Geometry check sheet. Reference: the model listing, model coordinates, mm. Face numbers are marked on the shaded views. A direction names the side the tool comes from. Round coordinates to 2 decimals unless told otherwise and drop trailing zeros. Order: outer loops, then holes, each group sorted by start corner. A loop starts at its lowest first (then second) coordinate and runs counter-clockwise, first axis right, second up.
(1) Cross-section at A-A on y = 20. Enter the section's corners in (x, z).
(2) Cross-section at B-B on x = 0. Enter the section's corners in (y, z).
(3) Set-up check for the marked faces 4, 5 and 6: record each of +Z, -Z, +X, -X, +Y, -Y from which the full face is reachable in a straight line by a thin tool's end or side.
(4) Thickness scan on L1, parallel to Y at x = -17, z = 0; L2, parallel to X at y = 50, z = 0; L3, parallel to Z at x = -17.5, y = 20. Record the ranges inside material, lowest first.
(5) Cross-section at D-D on z = 17. Enter the section's corners in (x, y).
(6) Draft check along Z on the marked faces 1, 2 and 3. Enter one of: pulls with the +Z half, pulls with the -Z half, needs draft (parallel to the pull), parting line crosses it, or undercut.
(7) Gauge pin test, flat ends, axial feed: P1, Ø21.5, axis at x = -32.5, y = 43.5, coming from the +Z side; P2, Ø5, axis at y = 40, z = 0, coming from the -X side; P3, Ø22, axis at x = 5.5, y = -12, coming from the -Z side. Record the tip position at first contact, or that the pin passes through.
(8) Cross-section at C-C on y = 50. Enter the section's corners in (x, z), and give its area (3 significant figures).
from build123d import *

# Parameters (mm, degrees)
SKETCH_1_W             = 40
SKETCH_1_H             = 40
EXTRUDE_1_DEPTH        = 60
SKETCH_2_R             = 15.1
CUT_EXTRUDE_1_DEPTH    = 50
SKETCH_3_R             = 2.5
EXTRUDE_2_DEPTH        = 5
SKETCH_4_R             = 1.5
CUT_EXTRUDE_2_DEPTH    = 75.833147735
PATTERN_LINEAR_1_COUNT = 2
PATTERN_LINEAR_1_PITCH = 20
SKETCH_5_W             = 8
SKETCH_5_H             = 14
EXTRUDE_3_DEPTH        = 27
FILLET_1_R             = 7
CUT_EXTRUDE_3_REACH    = 88.076
SKETCH_6_R             = 4
FILLET_2_R             = 20


with BuildPart() as part:
    # 草圖1 → 填料-伸長1 (new body)
    with BuildSketch(Plane(origin=(0, 0, 0), x_dir=(1, 0, 0), z_dir=(0, 1, 0))):
        Rectangle(SKETCH_1_W, SKETCH_1_H)
    extrude(amount=EXTRUDE_1_DEPTH)

    # 草圖2 → 除料-伸長1 (cut)
    with BuildSketch(Plane(origin=(0, 60, 0), x_dir=(1, 0, 0), z_dir=(0, 1, 0))):
        with Locations(Location((0, 0, 0), (0, 0, 270))):
            Circle(SKETCH_2_R)
    extrude(amount=-CUT_EXTRUDE_1_DEPTH, mode=Mode.SUBTRACT)

    # 草圖3 → 填料-伸長2 (add)
    with BuildSketch(Plane.XY.offset(20)):
        with BuildLine():
            Line((-20, 0), (20, 0))
            ThreePointArc((20, 0), (0, -20), (-20, 0))
        make_face()
        with Locations((0, -8)):
            Circle(SKETCH_3_R, mode=Mode.SUBTRACT)
    extrude(amount=-EXTRUDE_2_DEPTH)

    # 草圖4 → 除料-伸長2 (cut, through all)
    with BuildSketch(Plane(origin=(20, 0, 0), x_dir=(0, 0, -1), z_dir=(1, 0, 0))):
        with Locations((0, 20)):
            Circle(SKETCH_4_R)
    cut_extrude_2 = extrude(amount=-CUT_EXTRUDE_2_DEPTH, mode=Mode.SUBTRACT)

    # 直線複製排列1: 除料-伸長2 ×2
    with Locations(*[(0, i * PATTERN_LINEAR_1_PITCH, 0) for i in range(1, PATTERN_LINEAR_1_COUNT)]):
        add(cut_extrude_2, mode=Mode.SUBTRACT)

    # 草圖5 → 填料-伸長3 (add)
    with BuildSketch(Plane.ZY.offset(20)):
        with Locations((-16, 53)):
            Rectangle(SKETCH_5_W, SKETCH_5_H)
    extrude(amount=EXTRUDE_3_DEPTH)

    # 圓角1
    fillet_1_edges = [part.edges().sort_by_distance(p)[0] for p in [
        (-47, 46, -16),
        (-47, 60, -16),
    ]]
    fillet(fillet_1_edges, radius=FILLET_1_R - 0.0001)  # a hair under: the kernel refuses the full size

    # 草圖6 → 除料-伸長3 (cut, up to next)
    with BuildSketch(Plane(origin=(0, 0, -20), x_dir=(-1, 0, 0), z_dir=(0, 0, -1)), mode=Mode.PRIVATE) as cut_extrude_3_sk1:
        with Locations((40, 53)):
            Circle(SKETCH_6_R)
    cut_extrude_3_tool1 = extrude(cut_extrude_3_sk1.sketch, amount=-CUT_EXTRUDE_3_REACH, mode=Mode.PRIVATE) & part.part
    add(cut_extrude_3_tool1.solids().sort_by_distance((-40, 53, -20))[0], mode=Mode.SUBTRACT)

    # 圓角2
    fillet_2_edges = [part.edges().sort_by_distance(p)[0] for p in [
        (-20, 46, -16),
    ]]
    fillet(fillet_2_edges, radius=FILLET_2_R)


solid = part.part
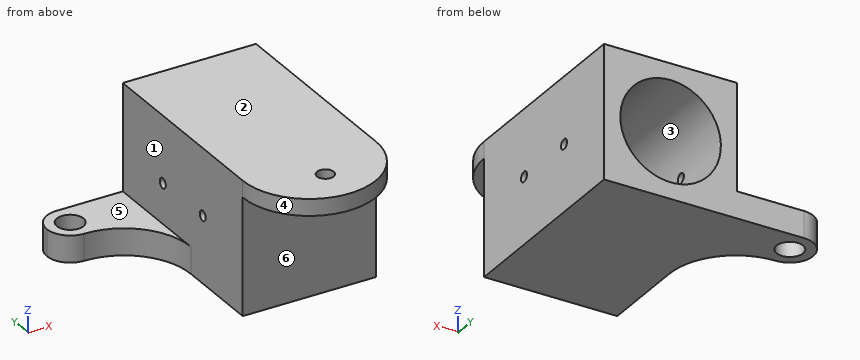
Found:
1. outline: (-20, -20) - (20, -20) - (20, -1.5) - (15.03, -1.5) arc R15.1 cw to (-15.03, -1.5) - (-20, -1.5) - close; (-20, 1.5) - (-15.03, 1.5) arc R15.1 cw to (15.03, 1.5) - (20, 1.5) - (20, 20) - (-20, 20) - close
2. outline: (-20, 15) - (-10.5, 15) - (-10.5, 20) - (-20, 20) - close; (-5.5, 15) - (0, 15) - (0, -20) - (60, -20) - (60, -15.1) - (10, -15.1) - (10, 15.1) - (60, 15.1) - (60, 20) - (-5.5, 20) - close
3. face 4: +Z, -Z, -Y
3. face 5: +Z, -X, +Y, -Y
3. face 6: -Z, +X, -X, -Y
4. L1: y = 0 to 18.5, 21.5 to 38.5, 41.5 to 60
4. L2: x = -20 to -15.1, 15.1 to 20
4. L3: z = -20 to -1.5, 1.5 to 20
5. outline: (-20, 0) arc R20 ccw to (20, 0) - (20, 60) - (-20, 60) - close; hole circle Ø5 at (0, -8)
6. face 1: needs draft
6. face 2: pulls with the +Z half
6. face 3: undercut
7. P1: stops at z = -12
7. P2: stops at x = -20
7. P3: stops at z = 15
8. outline: (-46.32, -20) - (-42.65, -20) - (-42.65, -12) - (-46.32, -12) - close; (-37.35, -20) - (20, -20) - (20, 20) - (-20, 20) - (-20, -12) - (-37.35, -12) - close; hole circle Ø30.2 at (0, 0)
8. area: 1,050 mm2
